Part model, mm, in its own coordinate system. A direction names the side the tool comes from. Round coordinates to 2 decimals unless told otherwise and drop trailing zeros. Order: outer loops, then holes, each group sorted by start corner. A loop starts at its lowest first (then second) coordinate and runs counter-clockwise, first axis right, second up. Notation, with made-up numbers: (55, 75.5) -> (61, 75.5) arc R15 ccw to (61, 96.5) -> close; hole circle Ø4 at (-29.5, 46). An arc over 180 degrees is marked (long way). Use CSV: the item, a comma, the result in double quotes.
Autodesk Inventor part; units mm, degrees
ref_plane "YZ Plane" through (0, 0, 0) normal (1, 0, 0) x (0, 1, 0)
ref_plane "XZ Plane" through (0, 0, 0) normal (0, 1, 0) x (-1, 0, 0)
ref_plane "XY Plane" through (0, 0, 0) normal (0, 0, 1) x (1, 0, 0)
sketch "Sketch1" plane through (0, 0, 0) normal (0, 1, 0) x (-1, 0, 0)
  circle A0 centre (0, 0) radius 19.05
  circle A1 centre (0, 0) radius 24.13
  line L0 (25.4, 25.4) -> (-25.4, 25.4)
  line L1 (-25.4, 25.4) -> (-25.4, -25.4)
  line L2 (-25.4, -25.4) -> (25.4, -25.4)
  line L3 (25.4, -25.4) -> (25.4, 25.4)
  line L4 (-25.4, -25.4) -> (-12.1092, -25.4) construction
  circle A2 centre (-20.32, -20.32) radius 3.175
  circle A3 centre (-20.32, 20.32) radius 3.175
  circle A4 centre (20.32, -20.32) radius 3.175
  circle A5 centre (20.32, 20.32) radius 3.175
  dimension "d10" = 50.8
  dimension "d11" = 50.8
  dimension "d20" = 6.35
extrude "Extrusion1" add sketch "Sketch1" along normal blind 50.8 contours A1
extrude "Extrusion3" add sketch "Sketch1" along normal blind 6.35 contours A1 | L3 L2 L1 L0 | A2 | A3 | A4 | A5
extrude "Extrusion5" cut sketch "Sketch1" along normal blind 6.35 contours A2 | A3 | A4 | A5
properties part number "Cylinders"
(1) Probe probe 1 along Z at (x, y) = (20.32, 3) (3 decimals); probe 2 along Z at (x, y) = (20, 4). List the from-to ranges inside material, lowest first. Write a range as [from, to].
Reply:
probe 1,"[-25.4, -23.495], [-17.145, 17.145], [23.495, 25.4]"
probe 2,"[-25.4, -23.48], [-17.16, 17.16], [23.48, 25.4]"
(2) Drop flat-ended pins along their axis: P1, Ø5, axis at y = 37.5, z = 0, coming from the -X side; P2, Ø1, axis at y = 28.5, z = 7, coming from the -X side; P3, Ø7.5, axis at x = -20.32, z = -20.32, coming from the +Y side; P4, Ø4, axis at x = 20.32, z = -20.32, coming from the -Y side (3 decimals). Give the stop position or say it passes through.
Reply:
P1,"x = -24.13"
P2,"x = -23.24"
P3,"y = 6.35"
P4,"through"
(3) Cut at C-C, the plane y = 27.5. Give the cut face in (x, z), then the cut area to 3 significant figures.
Reply:
outline,"circle Ø48.26 at (0, 0); hole circle Ø38.1 at (0, 0)"
area,"689 mm2"
(4) Cut at B-B, the plane z = 0. Give the cut face in (x, y), then the cut area to 3 significant figures.
Reply:
outline,"(-25.4, 0) -> (-19.05, 0) -> (-19.05, 50.8) -> (-24.13, 50.8) -> (-24.13, 6.35) -> (-25.4, 6.35) -> close; (19.05, 0) -> (25.4, 0) -> (25.4, 6.35) -> (24.13, 6.35) -> (24.13, 50.8) -> (19.05, 50.8) -> close"
area,"532 mm2"
(5) Which spindle directions (+Z, -Z, +X, -X, +Y, -Y) get a long thin tool onto all of the face, cutting with end or side? Do faces 1 (the face through (9.5, 6.35, -22.5)), 2 (the face through (0, 3, 25.4)). Say none if no direction does.
Reply:
face 1,"+Y"
face 2,"+Z, +X, -X, +Y, -Y"
(6) Cut at A-A, the plane x = 0. Give the cut face in (y, z), then the cut area to 3 significant figures.
Reply:
outline,"(0, -25.4) -> (6.35, -25.4) -> (6.35, -24.13) -> (50.8, -24.13) -> (50.8, -19.05) -> (0, -19.05) -> close; (0, 19.05) -> (50.8, 19.05) -> (50.8, 24.13) -> (6.35, 24.13) -> (6.35, 25.4) -> (0, 25.4) -> close"
area,"532 mm2"
(7) Cut at D-D, the plane z = 20.32. Give the cut face in (x, y) (3 decimals).
Reply:
outline,"(-25.4, 0) -> (-23.495, 0) -> (-23.495, 6.35) -> (-25.4, 6.35) -> close; (-17.145, 0) -> (17.145, 0) -> (17.145, 6.35) -> (13.014, 6.35) -> (13.014, 50.8) -> (-13.014, 50.8) -> (-13.014, 6.35) -> (-17.145, 6.35) -> close; (23.495, 0) -> (25.4, 0) -> (25.4, 6.35) -> (23.495, 6.35) -> close"
